Geometry: final body of the model. Coordinates: model frame, mm. A direction names the side the tool comes from. Coordinates: 2 decimals unless noted, no trailing zeros. Loops run counter-clockwise (first coordinate to the right, second up) from the corner with the lowest first, then second, coordinate; pieces in that order, holes last. Notation, with made-up numbers: (80, 62) -> (108, 62) arc R15 ccw to (108, 88) -> close; hole circle Ø3 at (-21, 41). An arc over 180 degrees is marked (long way). One line per item, written item: value. Start each with the question number.
from build123d import *

# Parameters (mm, degrees)
SKETCH1_R                     = 2.25
BOSS_EXTRUDE1_DEPTH           = 6
CUT_EXTRUDE1_DEPTH            = 10
F_4_5_4_5_DIAMETER_HOLE_D     = 4.5
F_4_5_4_5_DIAMETER_HOLE_DEPTH = 10
F_4_5_4_5_DIAMETER_HOLE_TIP   = 1.351936393
F_3_0MM_DOWEL_HOLE1_D         = 3
SKETCH7_R                     = 2.25
CUT_EXTRUDE2_DEPTH            = 10


with BuildPart() as part:
    # Sketch1 → Boss-Extrude1 (new body)
    with BuildSketch(Plane.XY):
        with BuildLine():
            Line((-65.035663909, 1.711915541), (-29.013741643, 43.763540838))
            ThreePointArc((-29.013741643, 43.763540838), (15.528638553, 54.242344325), (32.891210702, 96.578735816))
            Line((32.891210702, 96.578735816), (27.09893981, 163.698257544))
            ThreePointArc((27.09893981, 163.698257544), (127.465162664, -0.583384595), (-65.035663909, 1.711915541))
        make_face()
        with Locations((-44.130722543, 16.588386381)):
            Circle(SKETCH1_R, mode=Mode.SUBTRACT)
        with Locations((7.160790579, -31.047531597)):
            Circle(SKETCH1_R, mode=Mode.SUBTRACT)
        with Locations((100.470270724, 97.551800763)):
            Circle(SKETCH1_R, mode=Mode.SUBTRACT)
        with Locations((49.178757602, 145.187718741)):
            Circle(SKETCH1_R, mode=Mode.SUBTRACT)
    extrude(amount=BOSS_EXTRUDE1_DEPTH)

    # Sketch2 → Cut-Extrude1 (cut)
    with BuildSketch(Plane.XY.offset(6)):
        with BuildLine():
            Line((59.918631336, 48.293162369), (36.232435894, 68.292265986))
            ThreePointArc((36.232435894, 68.292265986), (35.982665158, 71.251592696), (38.941991868, 71.501363433))
            Line((38.941991868, 71.501363433), (62.62818731, 51.502259816))
            ThreePointArc((62.62818731, 51.502259816), (62.877958047, 48.542933105), (59.918631336, 48.293162369))
        make_face()
        with BuildLine():
            Line((39.274395345, 23.842896106), (15.588199903, 43.841999723))
            ThreePointArc((15.588199903, 43.841999723), (15.338429166, 46.801326433), (18.297755877, 47.05109717))
            Line((18.297755877, 47.05109717), (41.983951319, 27.051993553))
            ThreePointArc((41.983951319, 27.051993553), (42.233722055, 24.092666842), (39.274395345, 23.842896106))
        make_face()
    extrude(amount=-CUT_EXTRUDE1_DEPTH, mode=Mode.SUBTRACT)

    # Ø4.5 (4.5) Diameter Hole
    with Locations(Plane(origin=(207.215806152, -96.41995806, 6), x_dir=(-0.650558884, -0.759455817, 0), z_dir=(0, 0, 1))):
        with Locations((80.500098125, -194.461558154), (77.690872648, -264.405165812), (-80.677949684, -277.202176468), (-77.868724207, -207.25856881)):
            Hole(F_4_5_4_5_DIAMETER_HOLE_D / 2, depth=F_4_5_4_5_DIAMETER_HOLE_DEPTH)
            with Locations((0, 0, -(F_4_5_4_5_DIAMETER_HOLE_DEPTH + F_4_5_4_5_DIAMETER_HOLE_TIP / 2))):  # 118° drill point
                Cone(0, F_4_5_4_5_DIAMETER_HOLE_D / 2, F_4_5_4_5_DIAMETER_HOLE_TIP, mode=Mode.SUBTRACT)

    # Ø3.0mm Dowel Hole1 (through all)
    with Locations(Plane(origin=(207.215806152, -96.41995806, 6), x_dir=(-0.650558884, -0.759455817, 0), z_dir=(0, 0, 1))):
        with Locations((-80.915811264, -296.794954316), (-84.945199209, -182.518931257), (25.216324899, -241.36407945), (83.328606401, -169.42446636)):
            Hole(F_3_0MM_DOWEL_HOLE1_D / 2)

    # Sketch7 → Cut-Extrude2 (cut)
    with BuildSketch(Plane.XY.offset(6)):
        with Locations((39.410270698, -26.198883172)):
            Circle(SKETCH7_R)
        with Locations((110.999824953, 57.374033532)):
            Circle(SKETCH7_R)
        with Locations((24.221154353, -13.187705491)):
            Circle(SKETCH7_R)
        with Locations((95.810708608, 70.385211214)):
            Circle(SKETCH7_R)
        with Locations((121.384198104, 66.422365269)):
            Circle(SKETCH7_R)
        with Locations((131.142581365, 77.814202528)):
            Circle(SKETCH7_R)
        with BuildLine():
            Line((41.803278926, 132.877815745), (45.238927964, 93.066293708))
            ThreePointArc((45.238927964, 93.066293708), (45.878980474, 90.841973124), (47.31335672, 89.025428586))
            Line((47.31335672, 89.025428586), (72.343619279, 67.584208031))
            ThreePointArc((72.343619279, 67.584208031), (76.708983142, 66.158757194), (80.803707486, 68.23758963))
            Line((80.803707486, 68.23758963), (99.019356241, 89.502352513))
            ThreePointArc((99.019356241, 89.502352513), (100.444807079, 93.867716376), (98.365974642, 97.962440721))
            Line((98.365974642, 97.962440721), (51.684414291, 137.95042043))
            ThreePointArc((51.684414291, 137.95042043), (45.040870621, 138.731415078), (41.803278926, 132.877815745))
        make_face()
        with BuildLine():
            Line((139.689194778, 75.494313025), (118.594383125, 50.868444691))
            ThreePointArc((118.594383125, 50.868444691), (116.218631729, 43.592838252), (119.683352457, 36.768297678))
            Line((119.683352457, 36.768297678), (137.105326674, 21.84442739))
            Line((137.105326674, 21.84442739), (157.179168696, 45.278426173))
            Line((157.179168696, 45.278426173), (139.689194778, 75.494313025))
        make_face()
        with BuildLine():
            Line((26.971727927, -56.090910074), (47.00482887, -32.704472013))
            ThreePointArc((47.00482887, -32.704472013), (53.829369443, -29.239751286), (61.104975883, -31.615502682))
            Line((61.104975883, -31.615502682), (77.970944185, -46.063091691))
            Line((77.970944185, -46.063091691), (19.420644617, -114.414115242))
            Line((19.420644617, -114.414115242), (26.971727927, -56.090910074))
        make_face()
        with BuildLine():
            Line((30.087133776, 18.254417116), (14.029920526, 32.00921693))
            ThreePointArc((14.029920526, 32.00921693), (11.691810194, 33.244719456), (9.049641571, 33.355043432))
            Line((9.049641571, 33.355043432), (-26.432830213, 26.881246485))
            ThreePointArc((-26.432830213, 26.881246485), (-31.148141992, 22.543928053), (-29.259257867, 16.421950176))
            Line((-29.259257867, 16.421950176), (4.064778412, -12.123815573))
            ThreePointArc((4.064778412, -12.123815573), (8.430142276, -13.549266411), (12.52486662, -11.470433974))
            Line((12.52486662, -11.470433974), (30.740515375, 9.794328908))
            ThreePointArc((30.740515375, 9.794328908), (32.165966213, 14.159692772), (30.087133776, 18.254417116))
        make_face()
    extrude(amount=-CUT_EXTRUDE2_DEPTH, mode=Mode.SUBTRACT)


solid = part.part
1. Section C-C on x = 56. Return the cut outline in (y, z), plus the area to 3 significant figures.
2. Section A-A on x = -10. Return the cut outline in (y, z), plus the area to 3 significant figures.
3. Section B-B on y = 116.5. Return the cut outline in (x, z), plus the area to 3 significant figures.
4. Draft query along Y for faces 4 (the face through (62, 31, 6)), 5 (the face through (98.825, 141.061, 2.958)), 6 (the face through (69.42, -38.74, 3.04)), 7 (the face through (116.21, 43.7, 3.04)). Return one class per face: released by +Y, released by -Y, zero draft, split by the parting line, or undercut.
5. Set-up query: faces 1 (the face through (53.72, -29.25, 3.04)), 2 (the face through (48.241, 58.153, 3.042)), 3 (the face through (30.036, 129.669, 2.958)). Return all of +Z, -Z, +X, -X, +Y, -Y with unobstructed straight access to the full face (end or side cutting, diameter ignored); none if empty.
6. Section D-D on z = 3.75. Count the separate pieces of the cut face and the enclosed holes in it, plus the area to 3 significant figures.
7. Line query: L1, parallel to Y at x = 96.5, z = 5.25; L2, parallel to X at y = -30, z = 1.5; L3, parallel to X at y = 60, z = 4.75. Output: solid intervals per line, ascending. Write a range as [from, to].
8. Pin query (flat end, axial travel): pin 1 Ø1.5 at (y, z) = (35, 3.5) entering from -X; pin 2 Ø1.5 at (y, z) = (62.5, 5) entering from -X; pin 3 Ø3 at (x, z) = (-5, 3.5) entering from +Y. Return the tip coordinate at first contact, or that it passes through.
Checks:
1. outline: (-29.31, 0) -> (51.6, 0) -> (51.6, 6) -> (-29.31, 6) -> close; (57.1, 0) -> (81.58, 0) -> (81.58, 6) -> (57.1, 6) -> close; (134.25, 0) -> (161.12, 0) -> (161.12, 6) -> (134.25, 6) -> close
1. area: 794 mm²
2. outline: (-47.93, 0) -> (-0.08, 0) -> (-0.08, 6) -> (-47.93, 6) -> close; (29.88, 0) -> (42.76, 0) -> (42.76, 6) -> (29.88, 6) -> close
2. area: 364 mm²
3. outline: (31.17, 0) -> (43.22, 0) -> (43.22, 6) -> (31.17, 6) -> close; (76.73, 0) -> (122.23, 0) -> (122.23, 6) -> (76.73, 6) -> close
3. area: 345 mm²
4. face 4: zero draft
4. face 5: released by +Y
4. face 6: released by -Y
4. face 7: undercut
5. face 1: +Z, -Z, -Y
5. face 2: +Z, -Z
5. face 3: +Z, -Z, -X
6. separate pieces: 1
6. enclosed holes: 17
6. area: 20,600 mm²
7. L1: [-35.2, 68.24], [72.53, 86.56], [99.56, 142.8]
7. L2: [-39.41, 5.17], [9.15, 50.7], [58.49, 103.11]
7. L3: [21.26, 46.05], [52.56, 126.42]
8. pin 1: x = -37.16
8. pin 2: x = 22.67
8. pin 3: y = 44.12
